```python
from build123d import *

# Parameters (mm, degrees)
SKETCH1_W           = 7
SKETCH1_H           = 7
BOSS_EXTRUDE1_DEPTH = 3
CUT_EXTRUDE1_DEPTH  = 7
CUT_EXTRUDE2_DEPTH  = 11
SKETCH4_R           = 1.8
CUT_EXTRUDE3_DEPTH  = 0.8


with BuildPart() as part:
    # Sketch1 → Boss-Extrude1 (new body)
    with BuildSketch(Plane(origin=(0, 0, 0), x_dir=(1, 0, 0), z_dir=(0, 1, 0))):
        with Locations((3.5, 3.5)):
            Rectangle(SKETCH1_W, SKETCH1_H)
    extrude(amount=BOSS_EXTRUDE1_DEPTH)

    # Sketch2 → Cut-Extrude1 (cut)
    with BuildSketch(Plane.XY):
        Polygon((0, 0), (0.7, 3), (0, 3), align=None)
        Polygon((7, 0), (6.3, 3), (7, 3), align=None)
    extrude(amount=-CUT_EXTRUDE1_DEPTH, mode=Mode.SUBTRACT)

    # Sketch3 → Cut-Extrude2 (cut)
    with BuildSketch(Plane(origin=(0, 0, 0), x_dir=(0, 0, -1), z_dir=(1, 0, 0))):
        Polygon((0, 0), (0.7, 3), (0, 3), align=None)
        Polygon((7, 3), (6.3, 3), (7, 0), align=None)
    extrude(amount=CUT_EXTRUDE2_DEPTH, mode=Mode.SUBTRACT)

    # Sketch4 → Cut-Extrude3 (cut)
    with BuildSketch(Plane.XZ):
        with Locations(Location((3.5, -3.5, 0), (0, 0, 270))):
            Circle(SKETCH4_R)
    extrude(amount=-CUT_EXTRUDE3_DEPTH, mode=Mode.SUBTRACT)


solid = part.part
```
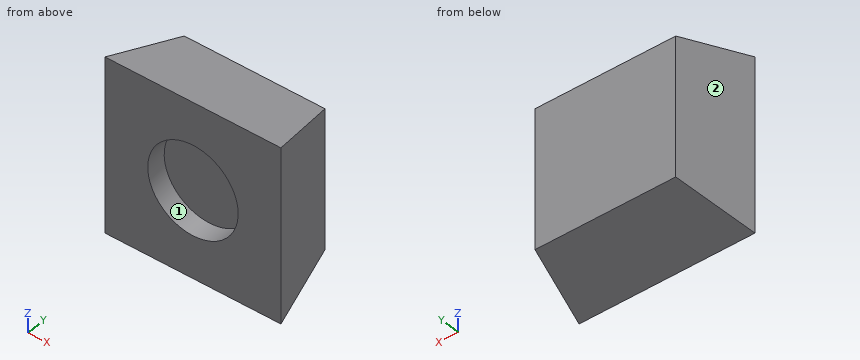
Geometry check sheet. Reference: the model listing, model coordinates, mm. Face numbers are marked on the shaded views. A direction names the side the tool comes from. Coordinates: 2 decimals unless noted, no trailing zeros. Order: outer loops, then holes, each group sorted by start corner. A loop starts at its lowest first (then second) coordinate and runs counter-clockwise, first axis right, second up. Notation, with made-up numbers: (-12.5, 5) - (-5.5, 5) arc R15 cw to (-5.5, 33) - close; hole circle Ø2 at (76, 49). An arc over 180 degrees is marked (long way). Use one line per item in the form item = value.
1. Section check A-A (z = -3.5). Record the boundary of the cut face in (x, y).
Here are the results:
outline = (0, 0) - (1.7, 0) - (1.7, 0.8) - (5.3, 0.8) - (5.3, 0) - (7, 0) - (6.3, 3) - (0.7, 3) - close
2. Scan lines: line 1 (X direction, y = 0.55, z = -3.5); line 2 (Y direction, x = 2, z = -3); line 3 (X direction, y = 0.2, z = -3.5). Record each from-to range of solid material in increasing order.
Here are the results:
line_1 = 0.13 to 1.7, 5.3 to 6.87
line_2 = 0.8 to 3
line_3 = 0.05 to 1.7, 5.3 to 6.95
3. Section check B-B (x = 3.5). Record the boundary of the cut face in (y, z).
Here are the results:
outline = (0, -7) - (3, -6.3) - (3, -0.7) - (0, 0) - (0, -1.7) - (0.8, -1.7) - (0.8, -5.3) - (0, -5.3) - close
4. Section check D-D (z = -1.5). Record the boundary of the cut face in (x, y).
Here are the results:
outline = (0, 0) - (7, 0) - (6.3, 3) - (0.7, 3) - close
5. Access from +Z, -Z, +X, -X, +Y, -Y to the whole of each face (thin tool, end or side, straight path). Record for the marked faces 1 and 2.
Here are the results:
face_1 = -Y
face_2 = +Z, -Z, -X, +Y
6. Section check C-C (y = 2.4). Record the boundary of the cut face in (x, z).
Here are the results:
outline = (0.56, -6.44) - (6.44, -6.44) - (6.44, -0.56) - (0.56, -0.56) - close
